Could you check a few things on this model? Use its own coordinates, in mm. Face numbers are marked on the shaded views. A direction names the side the tool comes from. Coordinates: 2 decimals unless noted, no trailing zeros. Write each loop counter-clockwise with the first axis right and the second up, starting at its lowest first coordinate (ties: lowest second). Pieces come first, ordered by that corner, then holes.
```python
from build123d import *

# Parameters (mm, degrees)
ESQUISSE1_R             = 50
ESQUISSE1_R_2           = 12.5
BOSS_EXTRU_1_DEPTH      = 4
ESQUISSE2_R             = 30
ESQUISSE2_R_2           = 12.5
BOSS_EXTRU_2_DEPTH      = 3
ENL_V_MAT_EXTRU_1_DEPTH = 23
ESQUISSE5_R             = 50
ESQUISSE5_R_2           = 40.5
BOSS_EXTRU_3_DEPTH      = 12.125


with BuildPart() as part:
    # Esquisse1 → Boss.-Extru.1 (new body)
    with BuildSketch(Plane.XY):
        Circle(ESQUISSE1_R)
        Circle(ESQUISSE1_R_2, mode=Mode.SUBTRACT)
    extrude(amount=BOSS_EXTRU_1_DEPTH)

    # Esquisse2 → Boss.-Extru.2 (add)
    with BuildSketch(Plane.XY.offset(4)):
        Circle(ESQUISSE2_R)
        Circle(ESQUISSE2_R_2, mode=Mode.SUBTRACT)
    extrude(amount=BOSS_EXTRU_2_DEPTH)

    # Esquisse4 → Enlèv. mat.-Extru.1 (cut)
    with BuildSketch(Plane(origin=(0, 0, 0), x_dir=(-1, 0, 0), z_dir=(0, 0, -1))):
        with BuildLine():
            Line((-4, 23.858960581), (-4, 34.340209667))
            ThreePointArc((-4, 34.340209667), (-5.945333747, 38.298620218), (-10.267605634, 39.176858916))
            ThreePointArc((-10.267605634, 39.176858916), (-28.637824638, 28.637824638), (-39.176858916, 10.267605634))
            ThreePointArc((-39.176858916, 10.267605634), (-38.298620218, 5.945333747), (-34.340209667, 4))
            Line((-34.340209667, 4), (-23.858960581, 4))
            ThreePointArc((-23.858960581, 4), (-21.014978286, 4.887608396), (-19.180733016, 7.235294118))
            ThreePointArc((-19.180733016, 7.235294118), (-14.495689014, 14.495689014), (-7.235294118, 19.180733016))
            ThreePointArc((-7.235294118, 19.180733016), (-4.887608396, 21.014978286), (-4, 23.858960581))
        make_face()
        with BuildLine():
            Line((4, 23.858960581), (4, 34.340209667))
            ThreePointArc((4, 34.340209667), (5.945333747, 38.298620218), (10.267605634, 39.176858916))
            ThreePointArc((10.267605634, 39.176858916), (28.637824638, 28.637824638), (39.176858916, 10.267605634))
            ThreePointArc((39.176858916, 10.267605634), (38.298620218, 5.945333747), (34.340209667, 4))
            Line((34.340209667, 4), (23.858960581, 4))
            ThreePointArc((23.858960581, 4), (21.014978286, 4.887608396), (19.180733016, 7.235294118))
            ThreePointArc((19.180733016, 7.235294118), (14.495689014, 14.495689014), (7.235294118, 19.180733016))
            ThreePointArc((7.235294118, 19.180733016), (4.887608396, 21.014978286), (4, 23.858960581))
        make_face()
        with BuildLine():
            Line((-23.858960581, -4), (-34.340209667, -4))
            ThreePointArc((-34.340209667, -4), (-38.298620218, -5.945333747), (-39.176858916, -10.267605634))
            ThreePointArc((-39.176858916, -10.267605634), (-28.637824638, -28.637824638), (-10.267605634, -39.176858916))
            ThreePointArc((-10.267605634, -39.176858916), (-5.945333747, -38.298620218), (-4, -34.340209667))
            Line((-4, -34.340209667), (-4, -23.858960581))
            ThreePointArc((-4, -23.858960581), (-4.887608396, -21.014978286), (-7.235294118, -19.180733016))
            ThreePointArc((-7.235294118, -19.180733016), (-14.495689014, -14.495689014), (-19.180733016, -7.235294118))
            ThreePointArc((-19.180733016, -7.235294118), (-21.014978286, -4.887608396), (-23.858960581, -4))
        make_face()
        with BuildLine():
            Line((23.858960581, -4), (34.340209667, -4))
            ThreePointArc((34.340209667, -4), (38.298620218, -5.945333747), (39.176858916, -10.267605634))
            ThreePointArc((39.176858916, -10.267605634), (28.637824638, -28.637824638), (10.267605634, -39.176858916))
            ThreePointArc((10.267605634, -39.176858916), (5.945333747, -38.298620218), (4, -34.340209667))
            Line((4, -34.340209667), (4, -23.858960581))
            ThreePointArc((4, -23.858960581), (4.887608396, -21.014978286), (7.235294118, -19.180733016))
            ThreePointArc((7.235294118, -19.180733016), (14.495689014, -14.495689014), (19.180733016, -7.235294118))
            ThreePointArc((19.180733016, -7.235294118), (21.014978286, -4.887608396), (23.858960581, -4))
        make_face()
    extrude(amount=-ENL_V_MAT_EXTRU_1_DEPTH, mode=Mode.SUBTRACT)

    # Esquisse5 → Boss.-Extru.3 (add)
    with BuildSketch(Plane(origin=(0, 0, 0), x_dir=(-1, 0, 0), z_dir=(0, 0, -1))):
        Circle(ESQUISSE5_R)
        Circle(ESQUISSE5_R_2, mode=Mode.SUBTRACT)
    extrude(amount=BOSS_EXTRU_3_DEPTH)


solid = part.part
```
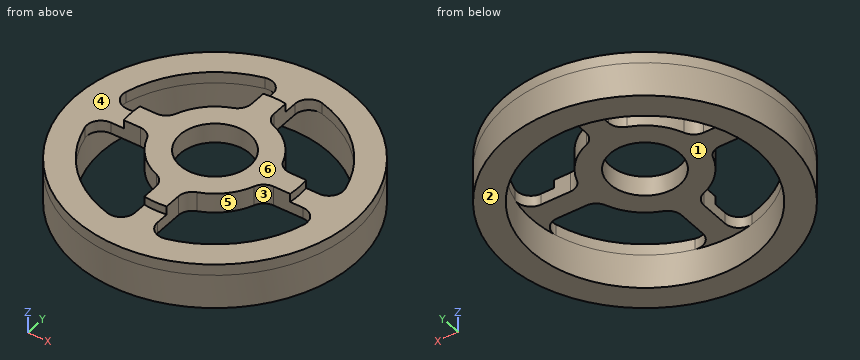
Item 1: I want a section at A-A, the plane y = 0. List the corners of the cut face in (x, z) for me (3 decimals).
Item 2: Which directions (+Z, -Z, +X, -X, +Y, -Y) give clear straight access to the entire face, cutting with the end or side of a thin tool? Please do the marked faces 1, 2, 3 and 4.
Item 3: If we mould it in two halves opening along X, with no side actions, what happens to the marked faces 5 and 6? For each: released by +X, released by -X, zero draft, split by the parting line, or undercut.
Item 4: I want a section at D-D, the plane y = 14. List the corners of the cut face in (x, z) for me (3 decimals).
Item 5: Will these pins go through, and if not, where does the flat tip stop? pin 1 Ø7.5 at (y, z) = (-27, 3.5) entering from -X; pin 2 Ø2 at (y, z) = (28.5, 4.5) entering from +X; pin 3 Ø3.5 at (y, z) = (31.5, 4.5) entering from -X.
Item 6: I want a section at C-C, the plane x = 28.5. List the corners of the cut face in (y, z) for me (3 decimals), then the cut area to 3 significant figures.
Item 7: If I drill on line 1 along Y through (x, z) = (0, 4.25); line 2 along Y through (x, z) = (0, 3.75); line 3 along Z through (x, y) = (-25.5, -0.5), over which ranges is the centre line in solid material (lowest first)?
Taken from the geometry:
1. outline: (-50, -12.125) - (-40.5, -12.125) - (-40.5, 0) - (-12.5, 0) - (-12.5, 7) - (-30, 7) - (-30, 4) - (-50, 4) - close; (12.5, 0) - (40.5, 0) - (40.5, -12.125) - (50, -12.125) - (50, 4) - (30, 4) - (30, 7) - (12.5, 7) - close
2. face 1: -Z
2. face 2: -Z, +X, -X, +Y, -Y
2. face 3: +Z, -Z
2. face 4: +Z
3. face 5: undercut
3. face 6: zero draft
4. outline: (-48, -12.125) - (-38.003, -12.125) - (-38.003, 4) - (-48, 4) - close; (-14.975, 0) - (14.975, 0) - (14.975, 7) - (-14.975, 7) - close; (38.003, -12.125) - (48, -12.125) - (48, 4) - (38.003, 4) - close
5. pin 1: stops at x = -44.27
5. pin 2: stops at x = 41.67
5. pin 3: stops at x = -40.13
6. outline: (-41.082, -12.125) - (-28.775, -12.125) - (-28.775, 4) - (-41.082, 4) - close; (-4, 0) - (4, 0) - (4, 7) - (-4, 7) - close; (28.775, -12.125) - (41.082, -12.125) - (41.082, 4) - (28.775, 4) - close
6. area: 453 mm2
7. line 1: y = -30 to -12.5, 12.5 to 30
7. line 2: y = -50 to -12.5, 12.5 to 50
7. line 3: z = 0 to 7
